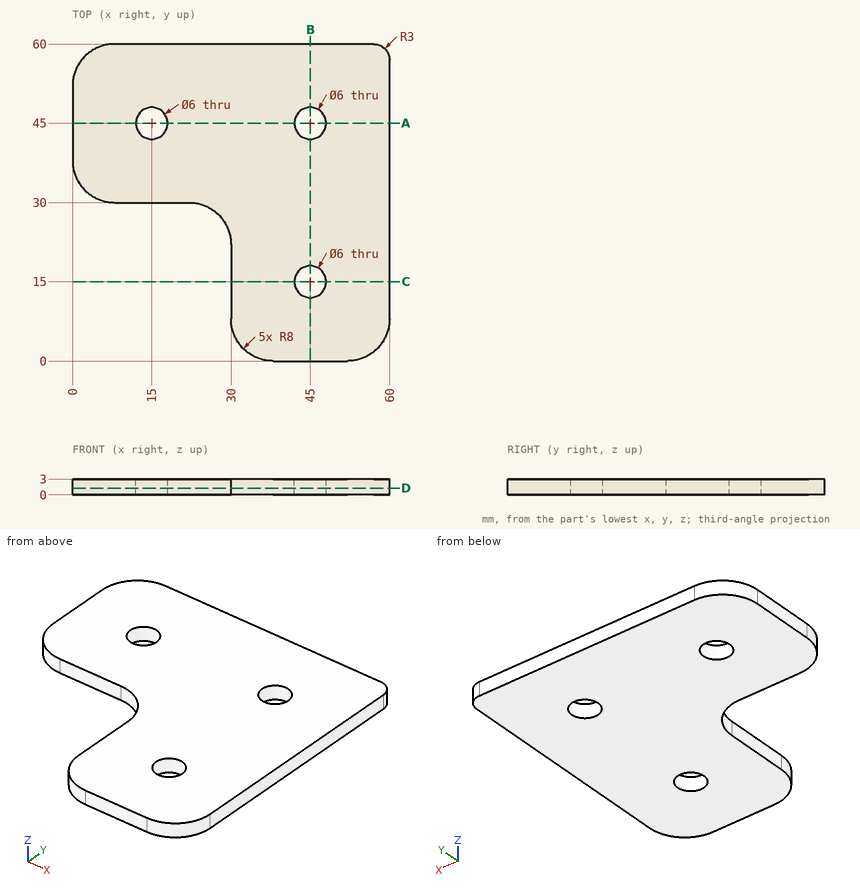
Design review of the part shown in the three views and the two pictorial views. Dimensions are in mm from the part's minimum x, y and z. Give positions to 0.01 mm unless a question says otherwise; leave off trailing zeros. Write each loop counter-clockwise with the first axis right and the second up, starting at its lowest first coordinate (ties: lowest second). Pieces come first, ordered by that corner, then holes.
(1) Add section A-A (y = 45). Give the boundary of the cut face in (x, z).
Checked values:
outline: (0, 0) - (12, 0) - (12, 3) - (0, 3) - close; (18, 0) - (42, 0) - (42, 3) - (18, 3) - close; (48, 0) - (60, 0) - (60, 3) - (48, 3) - close
(2) Add section C-C (y = 15). Give the boundary of the cut face in (x, z), and give its area (3 significant figures).
Checked values:
outline: (30, 0) - (42, 0) - (42, 3) - (30, 3) - close; (48, 0) - (60, 0) - (60, 3) - (48, 3) - close
area: 72.0 mm2
(3) Add section D-D (z = 1.25). Give the boundary of the cut face in (x, y), and give its area (3 significant figures).
Checked values:
outline: (0, 38) arc R8 ccw to (8, 30) - (22, 30) arc R8 cw to (30, 22) - (30, 8) arc R8 ccw to (38, 0) - (52, 0) arc R8 ccw to (60, 8) - (60, 57) arc R3 ccw to (57, 60) - (8, 60) arc R8 ccw to (0, 52) - close; hole circle Ø6 at (15, 45); hole circle Ø6 at (45, 15); hole circle Ø6 at (45, 45)
area: 2,570 mm2
(4) Wall thickness on line 1 along Y through (x, z) = (45, 2.35); line 2 along Y through (x, z) = (15, 1.55): over which ranges is each line inside the solid? List them lowest first.
Checked values:
line 1: y = 0 to 12, 18 to 42, 48 to 60
line 2: y = 30 to 42, 48 to 60
(5) Clearance check with flat-ended pins moving along their axes: pin 1 Ø1.5 at (y, z) = (17.5, 2) entering from -X; pin 2 Ø1.5 at (x, z) = (18, 2) entering from -Y; pin 3 Ø1 at (x, z) = (34.5, 1.5) entering from -Y. State where each tip first meets the part, or that it passes through.
Checked values:
pin 1: stops at x = 30
pin 2: stops at y = 30
pin 3: stops at y = 0.58
